Verification items for the finished model (mm, model axes). A direction names the side the tool comes from. Give positions to 0.01 mm unless a question says otherwise; leave off trailing zeros. Order: outer loops, then holes, each group sorted by start corner. A loop starts at its lowest first (then second) coordinate and runs counter-clockwise, first axis right, second up. Notation, with made-up numbers: (22, 42) - (28, 42) arc R23 ccw to (28, 76) - close; hole circle Ø8 at (87, -15.75). An arc over 180 degrees is marked (long way). Answer as a JSON object with one key per item and string values. Group by question number.
(1) Section check D-D (x = 20). Record the boundary of the cut face in (y, z).
(2) Section check A-A (z = 0). Record the boundary of the cut face in (x, y), then the cut area to 3 significant figures.
(3) Section check C-C (x = 33.5). Record the boundary of the cut face in (y, z).
(4) Thickness scan on line 1 (X direction, y = 8.5, z = 13.5); line 2 (X direction, y = 23.5, z = -16); line 3 (X direction, y = 21, z = 4.5). Record the ranges inside material, lowest first.
(5) Mould release check, pull along X, two halves, no side actions. Record for faces 1 (the face through (23.046, 22, 13)), 2 (the face through (62.009, -14.393, -4.533)), 3 (the face through (11.36, -6.35, 28.62)): +X half, -X half, draft (parallel to the pull), parting line (faces both ways), or undercut.
(6) Access from +Z, -Z, +X, -X, +Y, -Y to the whole of each face (thin tool, end or side, straight path). Record for faces 4 (the face through (100, 0, 0)), 5 (the face through (59.474, -3, -15)), 6 (the face through (31.04, 13.41, -21.04)).
(7) Depth check by flat-ended pin: pin 1 Ø6 at (x, z) = (36.5, 19.5) entering from +Y; pin 2 Ø4 at (x, y) = (11, -19) entering from +Z; pin 3 Ø1 at (x, z) = (25, 21.5) entering from +Y; pin 4 Ø10 at (y, z) = (11, 14.5) entering from -X. Enter the tip coordinate at first touch or a pass-through.
Autodesk Inventor part; units mm, degrees
ref_plane "YZ Plane" through (0, 0, 0) normal (1, 0, 0) x (0, 1, 0)
ref_plane "XZ Plane" through (0, 0, 0) normal (0, 1, 0) x (-1, 0, 0)
ref_plane "XY Plane" through (0, 0, 0) normal (0, 0, 1) x (1, 0, 0)
sketch "Эскиз1" plane through (0, 0, 0) normal (0, 0, 1) x (1, 0, 0)
  line L0 (0, 0) -> (100, 0)
  line L1 (100, 0) -> (100, 20.0896)
  line L2 (100, 20.0896) -> (39.2522, 20.0896)
  line L3 (39.2522, 20.0896) -> (39.2522, 24.9514)
  line L4 (39.2522, 24.9514) -> (23.0464, 24.9514)
  line L5 (23.0464, 24.9514) -> (23.0464, 29.3145)
  line L6 (23.0464, 29.3145) -> (0, 29.3145)
  line L7 (0, 29.3145) -> (0, 0)
  line L8 (59.4742, 20.0896) -> (59.4742, 15.0896)
  line L9 (59.4742, 15.0896) -> (64.4742, 15.0896)
  line L10 (64.4742, 15.0896) -> (64.4742, 20.0896)
  dimension "d0" = 100
  dimension "d2" = 5
  dimension "d3" = 5
revolve "Вращение1" add sketch "Эскиз1" angle 360 about axis through (0, 0, 0) along (1, 0, 0)
revolve "Вращение2" add sketch "Эскиз1" angle 360 about axis through (0, 0, 0) along (1, 0, 0) contours L10 L9 L8 L2
revolve "Вращение3" cut sketch "Эскиз1" angle 360 mid plane about axis through (0, 0, 0) along (1, 0, 0) contours L10 L9 L8 L2
properties part number "lab_4_1" material "Серебро"
Solutions:
{
 "1": {"outline": "circle Ø58.63 at (0, 0)"},
 "2": {"outline": "(0, -29.31) - (23.05, -29.31) - (23.05, -24.95) - (39.25, -24.95) - (39.25, -20.09) - (59.47, -20.09) - (59.47, -15.09) - (64.47, -15.09) - (64.47, -20.09) - (100, -20.09) - (100, 20.09) - (64.47, 20.09) - (64.47, 15.09) - (59.47, 15.09) - (59.47, 20.09) - (39.25, 20.09) - (39.25, 24.95) - (23.05, 24.95) - (23.05, 29.31) - (0, 29.31) - close", "area": "4,550 mm2"},
 "3": {"outline": "circle Ø49.9 at (0, 0)"},
 "4": {"line 1": "x = 0 to 59.47, 64.47 to 100", "line 2": "x = 0 to 23.05", "line 3": "x = 0 to 39.25"},
 "5": {"face 1": "+X half", "face 2": "undercut", "face 3": "draft"},
 "6": {"face 4": "+Z, -Z, +X, +Y, -Y", "face 5": "none", "face 6": "+X"},
 "7": {"pin 1": "stops at y = 18.72", "pin 2": "stops at z = 23.88", "pin 3": "stops at y = 13.47", "pin 4": "stops at x = 0"}
}
